Build history of the part. All positions in model axes, mm. Face numbers are marked on the shaded views. A direction names the side the tool comes from. Round coordinates to 2 decimals unless told otherwise and drop trailing zeros. Loops run counter-clockwise (first coordinate to the right, second up) from the corner with the lowest first, then second, coordinate; pieces in that order, holes last. Notation, with made-up numbers: (22.5, -36) - (46.5, -36) arc R17 ccw to (46.5, -8) - close; hole circle Ø10 at (-15.5, 19.25). An arc over 180 degrees is marked (long way). One line per question, with ' | ' between items. Start each with the question number.
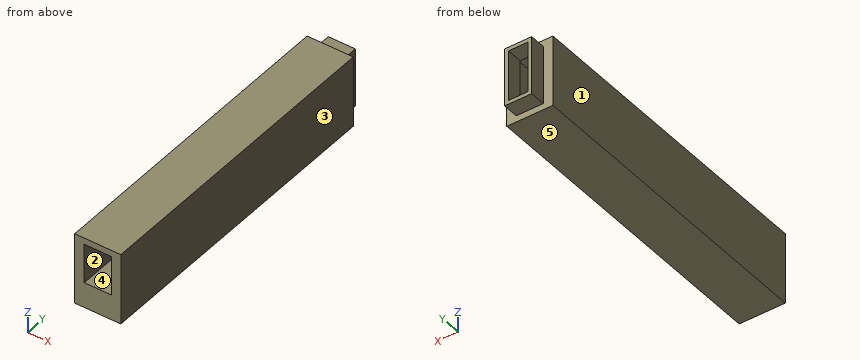
Autodesk Inventor part; units mm, degrees
ref_plane "YZ Plane" through (0, 0, 0) normal (1, 0, 0) x (0, 1, 0)
ref_plane "XZ Plane" through (0, 0, 0) normal (0, 1, 0) x (-1, 0, 0)
ref_plane "XY Plane" through (0, 0, 0) normal (0, 0, 1) x (1, 0, 0)
sketch "Sketch1" plane through (0, 0, 0) normal (0, 1, 0) x (-1, 0, 0)
  line L0 (5.3975, 11.7221) -> (-5.3975, 11.7221)
  line L1 (-5.3975, 11.7221) -> (-5.3975, -11.7221)
  line L2 (-5.3975, -11.7221) -> (5.3975, -11.7221)
  line L3 (5.3975, -11.7221) -> (5.3975, 11.7221)
  line L4 (5.3975, 11.7221) -> (-5.3975, -11.7221) construction
  line L5 (-5.3975, 11.7221) -> (5.3975, -11.7221) construction
  line L6 (9.2075, 14.2621) -> (-9.2075, 14.2621)
  line L7 (-9.2075, 14.2621) -> (-9.2075, -14.2621)
  line L8 (-9.2075, -14.2621) -> (9.2075, -14.2621)
  line L9 (9.2075, -14.2621) -> (9.2075, 14.2621)
  line L10 (9.2075, 14.2621) -> (-9.2075, -14.2621) construction
  line L11 (-9.2075, 14.2621) -> (9.2075, -14.2621) construction
  point P0 (0, 0)
  dimension "d0" = 10.795
  dimension "d1" = 23.4442
  dimension "d2" = 18.415
  dimension "d3" = 28.5242
extrude "Extrusion1" add sketch "Sketch1" along normal blind 127
sketch "Sketch2" plane through (0, 127, 0) normal (0, 1, 0) x (1, 0, 0)
  point P0 (0, 0)
sketch "Sketch3" plane through (0, 0, 0) normal (0, -1, 0) x (1, 0, 0)
  line L0 (5.3975, 11.7221) -> (5.3975, -11.7221)
  line L1 (-5.3975, 11.7221) -> (-5.3975, -11.7221)
  line L2 (5.3975, -11.7221) -> (-5.3975, -11.7221)
  line L3 (-5.3975, -11.7221) -> (-5.3975, -4.1021)
  line L4 (-5.3975, -4.1021) -> (5.3975, -4.1021)
  line L5 (5.3975, -4.1021) -> (5.3975, -11.7221)
  point P0 (0, 0)
  dimension "d6" = 7.62
extrude "Extrusion2" add sketch "Sketch3" against normal blind 127
sketch "Sketch4" plane through (0, 127, 0) normal (0, 1, 0) x (1, 0, 0)
  line L0 (-5.3975, 11.7221) -> (5.3975, 11.7221)
  line L1 (5.3975, 11.7221) -> (5.3975, -11.7221)
  line L2 (5.3975, -11.7221) -> (-5.3975, -11.7221)
  line L3 (-5.3975, -11.7221) -> (-5.3975, 11.7221)
  line L4 (-5.3975, 11.7221) -> (5.3975, -11.7221) construction
  line L5 (5.3975, 11.7221) -> (-5.3975, -11.7221) construction
  line L6 (-3.8735, 10.1981) -> (3.8735, 10.1981)
  line L7 (3.8735, 10.1981) -> (3.8735, -10.1981)
  line L8 (3.8735, -10.1981) -> (-3.8735, -10.1981)
  line L9 (-3.8735, -10.1981) -> (-3.8735, 10.1981)
  line L10 (-3.8735, 10.1981) -> (3.8735, -10.1981) construction
  line L11 (3.8735, 10.1981) -> (-3.8735, -10.1981) construction
  point P0 (0, 0)
  dimension "d9" = 10.795
  dimension "d10" = 23.4442
  dimension "d11" = 7.747
  dimension "d12" = 20.3962
extrude "Extrusion3" add sketch "Sketch4" along normal blind 6.35
properties part number "Bacon2"
1) Drop flat-ended pins along their axis: pin 1 (5 mm diameter, centred on x = 2.5, y = 130.5, fed in from +Z); pin 2 (3 mm diameter, centred on x = 2, z = -8, fed in from +Y); pin 3 (5 mm diameter, centred on y = 130, z = -3.5, fed in from +X); pin 4 (5.5 mm diameter, centred on x = -0.5, z = 2, fed in from -Y). Give the stop position or say it passes through.
2) Two-plate mould, pull along Z, no slides. Class the marked faces 3, 4 and 5: +Z half, -Z half, draft (parallel to the pull), parting line (faces both ways), or undercut.
3) Saw through at C-C on y = 90. Write the cut outline in (x, z).
4) Saw through at D-D on z = -5.25. Write the cut outline in (x, y), and give its area (3 significant figures).
5) Wall check: line 1 (X direction, y = 107, z = 8.5); line 2 (Z direction, x = -2.5, y = 63.5); line 3 (Y direction, x = 5.5, z = 2.25). Give the ranges that are in metal, low to high. Write a range as [from, to].
6) Tool access for the marked faces 1 and 2: list every direction of +Z, -Z, +X, -X, +Y, -Y with a clear straight run to the whole face (end or side of a thin tool).
Answer key:
1) pin 1: z = 11.72 | pin 2: y = 127 | pin 3: x = 5.4 | pin 4: through
2) face 3: draft | face 4: undercut | face 5: -Z half
3) outline: (-9.21, -14.26) - (9.21, -14.26) - (9.21, 14.26) - (-9.21, 14.26) - close; hole (-5.4, -4.1) - (5.4, -4.1) - (5.4, 11.72) - (-5.4, 11.72) - close
4) outline: (-9.21, 0) - (9.21, 0) - (9.21, 127) - (5.4, 127) - (5.4, 133.35) - (3.87, 133.35) - (3.87, 127) - (-3.87, 127) - (-3.87, 133.35) - (-5.4, 133.35) - (-5.4, 127) - (-9.21, 127) - close | area: 2,360 mm²
5) line 1: [-9.21, -5.4], [5.4, 9.21] | line 2: [-14.26, -4.1], [11.72, 14.26] | line 3: [0, 127]
6) face 1: +Z, -Z, -X, +Y, -Y | face 2: -Y
